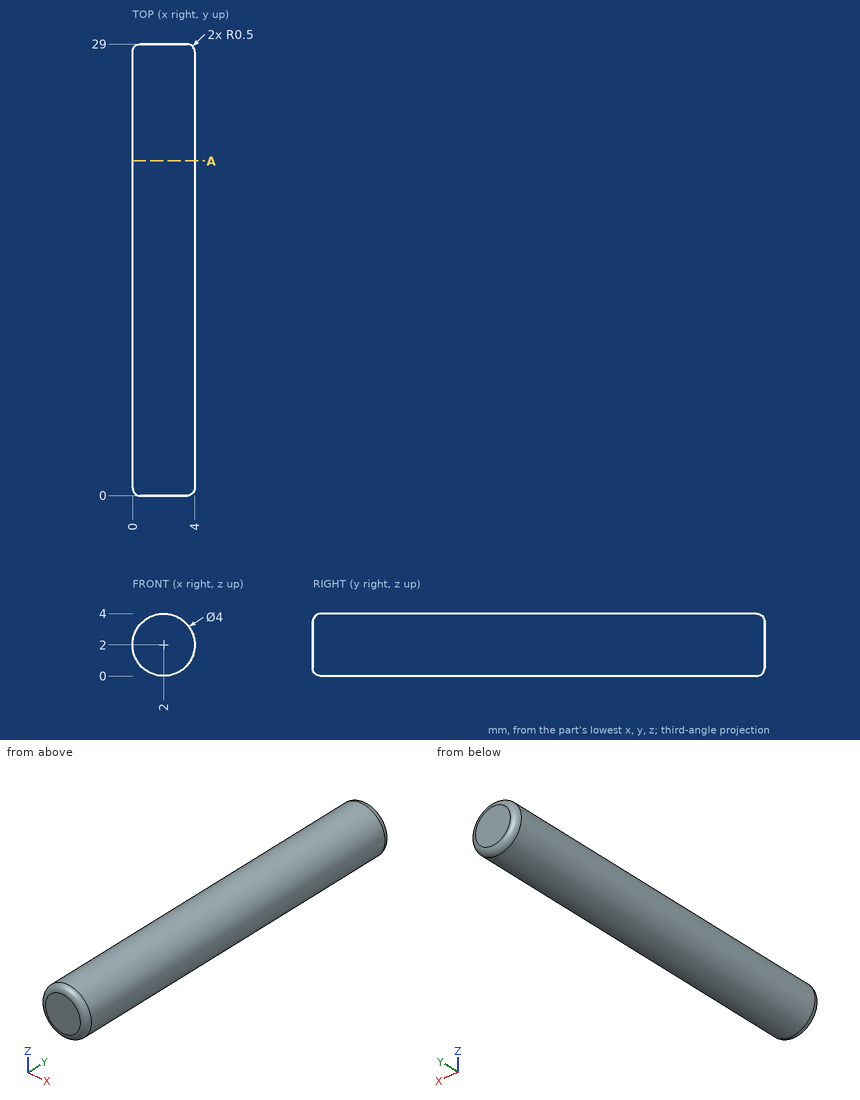
Job drawing, mm, ordinate dimensions from the low corner. One solid piece. Coordinates: 2 decimals unless noted, no trailing zeros. Write each loop counter-clockwise with the first axis right and the second up, starting at its lowest first coordinate (ties: lowest second). Pieces come first, ordered by that corner, then holes.
Item 1: Slice it at A-A (y = 21.5). Write the cut outline in (x, z).
Item 2: Probe line 1 (Y direction, x = 2.6, z = 0.45); line 2 (Z direction, x = 3.45, y = 18); line 3 (Z direction, x = 1.8, y = 26). List the from-to ranges inside material, lowest first.
Item 3: Pin check, flat tips, straight feed: pin 1 (1.5 mm diameter, centred on x = 2, z = 3, fed in from -Y); pin 2 (1.5 mm diameter, centred on y = 8.5, z = 0.5, fed in from +X); pin 3 (1.5 mm diameter, centred on y = 10.5, z = 1, fed in from +X). Stop position of each tip, or through.
Results found:
1. outline: circle Ø4 at (2, 2)
2. line 1: y = 0.03 to 28.97
2. line 2: z = 0.62 to 3.38
2. line 3: z = 0.01 to 3.99
3. pin 1: stops at y = 0
3. pin 2: stops at x = 3.85
3. pin 3: stops at x = 3.98
